Could you check a few things on this model? Use its own coordinates, in mm. A direction names the side the tool comes from. Round coordinates to 2 decimals unless told otherwise and drop trailing zeros. Write each loop counter-clockwise with the first axis right and the second up, starting at its lowest first coordinate (ties: lowest second). Pieces come first, ordered by that corner, then holes. Notation, with made-up numbers: (39, -4) - (44, -4) arc R28 ccw to (44, 30) - close; hole circle Ø8 at (13, -36.75). An arc over 180 degrees is marked (long way). Put each result on its own line as item: value.
from build123d import *

# Parameters (mm, degrees)
SKETCH_1_W          = 140
SKETCH_1_H          = 200
EXTRUDE_1_DEPTH     = 3
SKETCH_2_W          = 65
SKETCH_2_H          = 50
CUT_EXTRUDE_1_DEPTH = 10
SKETCH_4_W          = 3
SKETCH_4_H          = 55
EXTRUDE_4_DEPTH     = 18
CUT_EXTRUDE_2_REACH = 244.211
SKETCH_5_R          = 1.5
SKETCH_6_W          = 18
SKETCH_6_H          = 55
SKETCH_6_R          = 1.5
EXTRUDE_6_DEPTH     = 3


with BuildPart() as part:
    # 草图1 → 凸台-拉伸1 (new body)
    with BuildSketch(Plane.XY):
        with Locations((70, -100)):
            Rectangle(SKETCH_1_W, SKETCH_1_H)
    extrude(amount=EXTRUDE_1_DEPTH)

    # 草图2 → 切除-拉伸1 (cut)
    with BuildSketch(Plane(origin=(0, 0, 0), x_dir=(-1, 0, 0), z_dir=(0, 0, -1))):
        with Locations((-32.5, -175)):
            Rectangle(SKETCH_2_W, SKETCH_2_H)
    extrude(amount=-CUT_EXTRUDE_1_DEPTH, mode=Mode.SUBTRACT)

    # 草图4 → 凸台-拉伸4 (add)
    with BuildSketch(Plane.XY.offset(3)):
        with Locations((6.5, -54.5)):
            Rectangle(SKETCH_4_W, SKETCH_4_H)
    extrude(amount=EXTRUDE_4_DEPTH)

    # 草图5 → 切除-拉伸2 (cut, up to next)
    with BuildSketch(Plane.ZY.offset(-5), mode=Mode.PRIVATE) as cut_extrude_2_sk1:
        with Locations(Location((13, -76.16447412, 0), (0, 0, 270))):
            Circle(SKETCH_5_R)
    cut_extrude_2_tool1 = extrude(cut_extrude_2_sk1.sketch, amount=-CUT_EXTRUDE_2_REACH, mode=Mode.PRIVATE) & part.part
    # 草图5 → 切除-拉伸2 (cut, up to next)
    with BuildSketch(Plane.ZY.offset(-5), mode=Mode.PRIVATE) as cut_extrude_2_sk2:
        with Locations(Location((13, -36.16447412, 0), (0, 0, 270))):
            Circle(SKETCH_5_R)
    cut_extrude_2_tool2 = extrude(cut_extrude_2_sk2.sketch, amount=-CUT_EXTRUDE_2_REACH, mode=Mode.PRIVATE) & part.part
    add(cut_extrude_2_tool1.solids().sort_by_distance((5, -76.164474, 13))[0], mode=Mode.SUBTRACT)
    add(cut_extrude_2_tool2.solids().sort_by_distance((5, -36.164474, 13))[0], mode=Mode.SUBTRACT)

    # 草图6 → 凸台-拉伸6 (add)
    with BuildSketch(Plane(origin=(128, 0, 0), x_dir=(0, 0, -1), z_dir=(1, 0, 0))):
        with Locations((-12, -54.5)):
            Rectangle(SKETCH_6_W, SKETCH_6_H)
        with Locations(Location((-13, -76.16447412, 0), (0, 0, 270))):
            Circle(SKETCH_6_R, mode=Mode.SUBTRACT)
        with Locations(Location((-13, -36.16447412, 0), (0, 0, 270))):
            Circle(SKETCH_6_R, mode=Mode.SUBTRACT)
    extrude(amount=EXTRUDE_6_DEPTH)


solid = part.part
(1) If we mould it in two halves opening along X, with no side actions, what happens to faces 1 (the face through (69, -99, 0)), 2 (the face through (8, -55, 12)), 3 (the face through (131, -54, 12))? For each: pulls with the +X half, pulls with the -X half, needs draft (parallel to the pull), parting line crosses it, or undercut.
Values found:
face 1: needs draft
face 2: undercut
face 3: pulls with the +X half
(2) Imagine slicing it at B-B, the plane y = -58. List the corners of the cut face in (x, z) for me.
Values found:
outline: (0, 0) - (140, 0) - (140, 3) - (131, 3) - (131, 21) - (128, 21) - (128, 3) - (8, 3) - (8, 21) - (5, 21) - (5, 3) - (0, 3) - close
(3) Imagine slicing it at A-A, the plane z = 6.75. List the corners of the cut face in (x, y) for me, then the cut area to 3 significant figures.
Values found:
outline: (5, -82) - (8, -82) - (8, -27) - (5, -27) - close; (128, -82) - (131, -82) - (131, -27) - (128, -27) - close
area: 330 mm^2
(4) For faces 4 (the face through (128, -54, 12)), 5 (the face through (5, -55, 12)), which set-ups out of +Z, -Z, +X, -X, +Y, -Y let a thin tool reach every point of the face, with its end or its side?
Values found:
face 4: +Z, +Y, -Y
face 5: +Z, -X, +Y, -Y
(5) I'm going to push flat-ended pins straight in: pin 1 (0.9 mm diameter, centred on x = 6, z = 12.5, fed in from +Y); pin 2 (0.9 mm diameter, centred on x = 7, z = 11, fed in from -Y); pin 3 (5.5 mm diameter, centred on y = -53.5, z = 9, fed in from -X); pin 4 (8 mm diameter, centred on x = 49, z = 10.5, fed in from -Y). Where does each tip first touch, or does it pass through?
Values found:
pin 1: stops at y = -27
pin 2: stops at y = -82
pin 3: stops at x = 5
pin 4: passes through
(6) Imagine slicing it at D-D, the plane y = -88.5. List the corners of the cut face in (x, z) for me, then the cut area to 3 significant figures.
Values found:
outline: (0, 0) - (140, 0) - (140, 3) - (0, 3) - close
area: 420 mm^2
(7) Please list where these lines run through material, in increasing order: probe 1 along Y at (x, z) = (128.9, 13); probe 2 along X at (y, z) = (-33, 3.75); probe 3 along Z at (x, y) = (37.5, -74). Write a range as from..to.
Values found:
probe 1: y = -82..-77.66, -74.66..-37.66, -34.66..-27
probe 2: x = 5..8, 128..131
probe 3: z = 0..3
(8) Imagine slicing it at C-C, the plane x = 68. List the corners of the cut face in (y, z) for me, then the cut area to 3 significant figures.
Values found:
outline: (-200, 0) - (0, 0) - (0, 3) - (-200, 3) - close
area: 600 mm^2
